from build123d import *

# Parameters (mm, degrees)
F0_R     = 4
F1_DEPTH = 20
F2_R     = 0.325
F3_DEPTH = 10


with BuildPart() as f1:
    # F0 (on Top) → F1 (new body)
    with BuildSketch(Plane.XY):
        Circle(F0_R)
    extrude(amount=F1_DEPTH)

    # F2 (on face) → F3 (join)
    with BuildSketch(Plane(origin=(0, 0, 0), x_dir=(1, 0, 0), z_dir=(0, 0, -1))):
        with Locations((-1.75, 0)):
            Circle(F2_R)
        with Locations((1.75, 0)):
            Circle(F2_R)
    extrude(amount=F3_DEPTH)


solid = f1.part
The model under review builds one solid part; all positions refer to its coordinate system, in mm. Round coordinates to 2 decimals unless told otherwise and drop trailing zeros. Loops run counter-clockwise (first coordinate to the right, second up) from the corner with the lowest first, then second, coordinate; pieces in that order, holes last. Notation, with made-up numbers: M 24,75 L 71,75 A26 cw 71,114 Z; hole C 74,22.5 d8. An arc over 180 degrees is marked long. Answer as a JSON object with one key per item and string values.
Item 1: We need section A-A, the plane y = 0. State the section outline as (x, z) points (3 decimals).
Check sheet entries:
{"outline": "M -4,0 L -2.075,0 L -2.075,-10 L -1.425,-10 L -1.425,0 L 1.425,0 L 1.425,-10 L 2.075,-10 L 2.075,0 L 4,0 L 4,20 L -4,20 Z"}
Item 2: For line 1 along X through (y, z) = (0, -4.25) (3 decimals); line 2 along Z through (x, y) = (-2, 1); line 3 along Y through (x, z) = (-3, 1.5), list the stretches that pass through material, from the lowest coordinate up.
Check sheet entries:
{"line 1": "-2.075 to -1.425, 1.425 to 2.075", "line 2": "0 to 20", "line 3": "-2.65 to 2.65"}
Item 3: We need section B-B, the plane z = -8. State the section outline as (x, y) points (3 decimals).
Check sheet entries:
{"outline": "C -1.75,0 d0.65; C 1.75,0 d0.65"}
Item 4: Clearance check with flat-ended pins moving along their axes: P1, Ø3, axis at x = 1, z = -3, coming from the +Y side (3 decimals); P2, Ø1.5, axis at x = 0.5, y = 0, coming from the -Z side. State where each tip first meets the part, or that it passes through.
Check sheet entries:
{"P1": "y = 0.325", "P2": "z = 0"}
Item 5: We need section D-D, the plane z = 18. State the section outline as (x, y) points.
Check sheet entries:
{"outline": "C 0,0 d8"}
Item 6: We need section C-C, the plane x = 0. State the section outline as (y, z) points.
Check sheet entries:
{"outline": "M -4,0 L 4,0 L 4,20 L -4,20 Z"}
